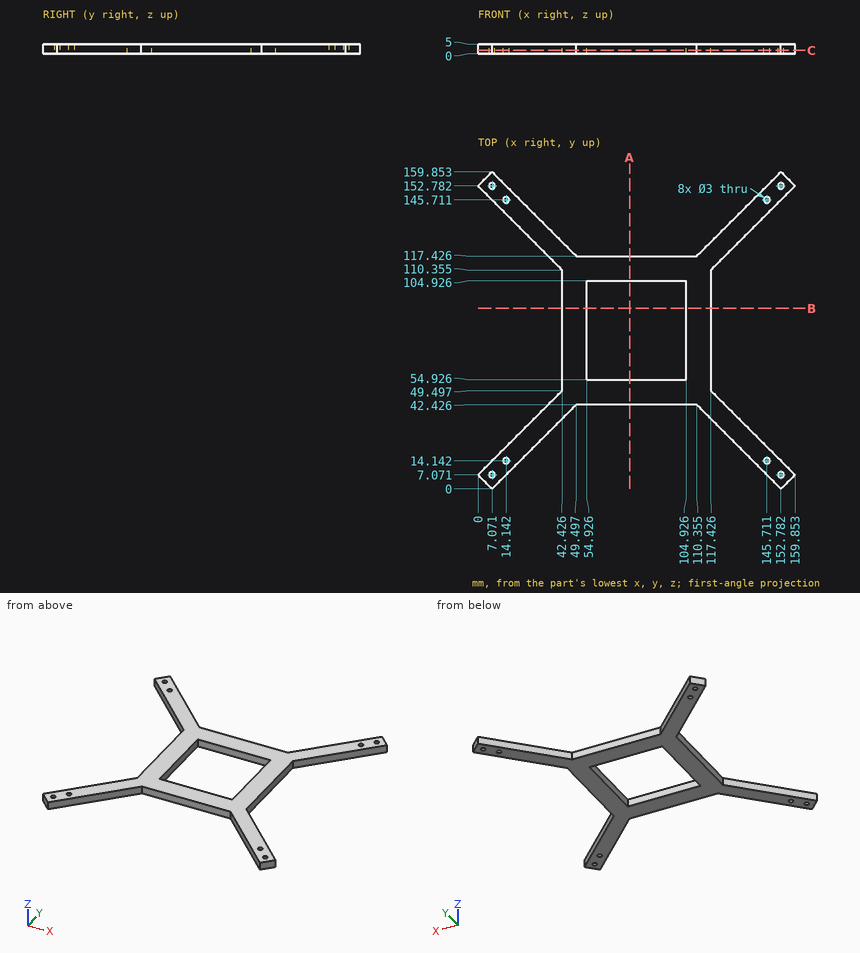
Can you work these out from the drawing? Everything is in mm from the part's minimum corner. Give positions to 0.01 mm unless a question says otherwise; leave off trailing zeros. Order: outer loops, then holes, each group sorted by start corner. A loop starts at its lowest first (then second) coordinate and runs counter-clockwise, first axis right, second up.
1. Suppose I cut it at C-C (z = 1.75). Give the number of separate pieces and of enclosed holes in the cut face, plus the area to 3 significant figures.
2. I need wall thicknesses on L1, parallel to X at y = 72, z = 4.75; L2, parallel to Y at x = 14.5, z = 2.65 (1 decimal). Which ranges of each line are inside material? Lowest first, please.
3. Will these pins go through, and if not, where does the flat tip stop? P1, Ø3, axis at x = 63.5, z = 2.5, coming from the +Y side; P2, Ø1.5, axis at x = 90.5, z = 3, coming from the -Y side; P3, Ø3, axis at x = 35, z = 1, coming from the -Y side; P4, Ø2.5, axis at x = 7.07, y = 7.07, coming from the -Z side (3 decimals).
4. Suppose I cut it at A-A (x = 76.5). List the corners of the cut face in (y, z) for me.
Solved:
1. separate pieces: 1
1. enclosed holes: 9
1. area: 5,370 mm2
2. L1: x = 42.43 to 54.93, 104.93 to 117.43
2. L2: y = 7.4 to 12.7, 15.6 to 21.6, 138.3 to 144.3, 147.2 to 152.4
3. P1: stops at y = 117.43
3. P2: stops at y = 42.43
3. P3: stops at y = 26.43
3. P4: passes through
4. outline: (42.43, 0) - (54.93, 0) - (54.93, 5) - (42.43, 5) - close; (104.93, 0) - (117.43, 0) - (117.43, 5) - (104.93, 5) - close
